```python
from build123d import *

# Parameters (mm, degrees)
CROQUIS2_W              = 40
CROQUIS2_H              = 60
SALIENTE_EXTRUIR1_DEPTH = 30
CROQUIS3_W              = 50
CROQUIS3_H              = 30
SALIENTE_EXTRUIR2_DEPTH = 20
CROQUIS4_W              = 50
CROQUIS4_H              = 30
SALIENTE_EXTRUIR3_DEPTH = 20


with BuildPart() as part:
    # Croquis2 → Saliente-Extruir1 (new body)
    with BuildSketch(Plane.XY):
        Rectangle(CROQUIS2_W, CROQUIS2_H)
    extrude(amount=SALIENTE_EXTRUIR1_DEPTH)

    # Croquis3 → Saliente-Extruir2 (add)
    with BuildSketch(Plane(origin=(20, 0, 0), x_dir=(0, 0, -1), z_dir=(1, 0, 0))):
        with Locations((-25, -15)):
            Rectangle(CROQUIS3_W, CROQUIS3_H)
    extrude(amount=SALIENTE_EXTRUIR2_DEPTH)

    # Croquis4 → Saliente-Extruir3 (add)
    with BuildSketch(Plane.ZY.offset(20)):
        with Locations((25, -15)):
            Rectangle(CROQUIS4_W, CROQUIS4_H)
    extrude(amount=SALIENTE_EXTRUIR3_DEPTH)


solid = part.part
```
CAD build for the part. Positions are in the model's coordinates, mm. A direction names the side the tool comes from. Coordinates: 2 decimals unless noted, no trailing zeros. Order: outer loops, then holes, each group sorted by start corner. A loop starts at its lowest first (then second) coordinate and runs counter-clockwise, first axis right, second up. Notation, with made-up numbers: (3, 6) - (59, 6) arc R32 ccw to (59, 37) - close; hole circle Ø10 at (-2.75, 35). An arc over 180 degrees is marked (long way). Use a Markdown table: item, result. Add a question column.
(1) Drill centre lines: line 1 along X through (y, z) = (-13, 37); line 2 along X through (y, z) = (6, 20.5); line 3 along Y through (x, z) = (-25.5, 20). Where is each one in solid material? Low to high. Write a range as [from, to].
(2) Saw through at B-B (y = -25). Give the cut face in (x, z), then the cut area to 3 significant figures.
(3) Saw through at D-D (x = 21). Give the cut face in (y, z), then the cut area to 3 significant figures.
(4) Which spindle directions (+Z, -Z, +X, -X, +Y, -Y) get a long thin tool onto all of the face, cutting with end or side? Do faces 1 (the face through (20, -15, 40)), 2 (the face through (-20, 15, 15)), 3 (the face through (30, 0, 25)), 4 (the face through (40, -15, 25)). Say none if no direction does.
(5) Saw through at C-C (z = 7). Give the cut face in (x, y), then the cut area to 3 significant figures.
(6) Flat gauge pins, fed straight in: pin 1 (16 mm diameter, centred on x = -30.5, z = 24, fed in from +Y); pin 2 (12 mm diameter, centred on x = -23, y = 15, fed in from +Z); pin 3 (24 mm diameter, centred on y = 22, z = 17.5, fed in from +X). Where does each tip first touch, or does it go through?
(7) Saw through at A-A (z = 31). Give the cut face in (x, y).
Solved:
| question | item | result |
|---|---|---|
| 1 | line 1 | x = [-40, -20], [20, 40] |
| 1 | line 2 | x = [-20, 20] |
| 1 | line 3 | y = [-30, 0] |
| 2 | outline | (-40, 0) - (40, 0) - (40, 50) - (20, 50) - (20, 30) - (-20, 30) - (-20, 50) - (-40, 50) - close |
| 2 | area | 3,200 mm² |
| 3 | outline | (-30, 0) - (0, 0) - (0, 50) - (-30, 50) - close |
| 3 | area | 1,500 mm² |
| 4 | face 1 | +Z, +Y, -Y |
| 4 | face 2 | +Z, -Z, -X, +Y |
| 4 | face 3 | +Z, -Z, +X, +Y |
| 4 | face 4 | +Z, -Z, +X, +Y, -Y |
| 5 | outline | (-40, -30) - (40, -30) - (40, 0) - (20, 0) - (20, 30) - (-20, 30) - (-20, 0) - (-40, 0) - close |
| 5 | area | 3,600 mm² |
| 6 | pin 1 | stops at y = 0 |
| 6 | pin 2 | stops at z = 30 |
| 6 | pin 3 | stops at x = 20 |
| 7 | outline | (-40, -30) - (-20, -30) - (-20, 0) - (-40, 0) - close; (20, -30) - (40, -30) - (40, 0) - (20, 0) - close |
